Source: CAD feature listing. Evaluate the final solid. Frame: model axes, mm. Face numbers are marked on the shaded views. A direction names the side the tool comes from. Coordinates: 2 decimals unless noted, no trailing zeros. Loops run counter-clockwise (first coordinate to the right, second up) from the corner with the lowest first, then second, coordinate; pieces in that order, holes last.
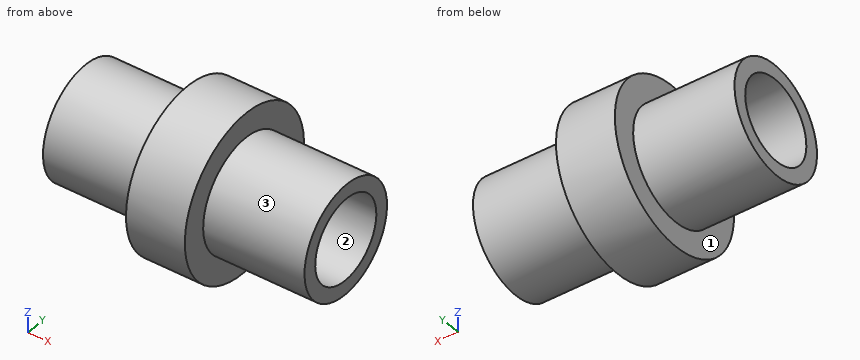
```python
from build123d import *

# Parameters (mm, degrees)
CUT_EXTRUDE1_DEPTH      = 44.767370257
CUT_EXTRUDE1_DEPTH_BACK = 44.767370257
SKETCH3_R               = 6.35


with BuildPart() as part:
    # Sketch2 → Revolve1 (revolve)
    with BuildSketch(Plane(origin=(0, 0, 0), x_dir=(1, 0, 0), z_dir=(0, 1, 0))):
        Polygon((-20.055735381, 8.5725), (-4.510240996, 8.5725), (-4.510240996, 12.3825), (4.510240996, 12.3825), (4.510240996, 8.5725), (20.055735381, 8.5725), (20.055735381, 0), (-20.055735381, 0), align=None)
    revolve(axis=Axis((20.055735381, 0, 0), (-1, 0, 0)))

    # Sketch3 → Cut-Extrude1 (cut, two sides: drawn at the far end of the back side and taken through both)
    with BuildSketch(Plane(origin=(20.055735381, 0, 0), x_dir=(0, 0, -1), z_dir=(1, 0, 0)).offset(-CUT_EXTRUDE1_DEPTH_BACK)):
        Circle(SKETCH3_R)
    extrude(amount=CUT_EXTRUDE1_DEPTH + CUT_EXTRUDE1_DEPTH_BACK, mode=Mode.SUBTRACT)


solid = part.part
```
Q1. First-contact query: pin 1 Ø3 at (x, y) = (14.5, -2.5) entering from +Z; pin 2 Ø10 at (x, z) = (-7, 8) entering from +Y; pin 3 Ø7.5 at (y, z) = (-5, -0.5) entering from -X; pin 4 Ø6 at (x, z) = (-12, -6.5) entering from -Y. Flat tips, straight axial feed; report the tip coordinate or a pass-through.
Q2. Section query A-A on y = 0. Return the cut outline in (x, z), then the cut area to 3 significant figures.
Q3. Material intervals for line 1 along Z through (x, y) = (-9, 0); line 2 along Y through (x, z) = (-1, 0), sorted ascending.
Q4. Section query D-D on y = 8. Return the cut outline in (x, z), then the cut area to 3 significant figures.
Q5. Reachability of the marked faces 1, 2 and 3 from +Z, -Z, +X, -X, +Y, -Y: full face, straight path, thin tool, end or side. Return the list, or none.
Resolved:
1. pin 1: stops at z = 8.51
1. pin 2: stops at y = 11.83
1. pin 3: stops at x = -20.06
1. pin 4: stops at y = -7.83
2. outline: (-20.06, -8.57) - (-4.51, -8.57) - (-4.51, -12.38) - (4.51, -12.38) - (4.51, -8.57) - (20.06, -8.57) - (20.06, -6.35) - (-20.06, -6.35) - close; (-20.06, 6.35) - (20.06, 6.35) - (20.06, 8.57) - (4.51, 8.57) - (4.51, 12.38) - (-4.51, 12.38) - (-4.51, 8.57) - (-20.06, 8.57) - close
2. area: 247 mm2
3. line 1: z = -8.57 to -6.35, 6.35 to 8.57
3. line 2: y = -12.38 to -6.35, 6.35 to 12.38
4. outline: (-20.06, -3.08) - (-4.51, -3.08) - (-4.51, -9.45) - (4.51, -9.45) - (4.51, -3.08) - (20.06, -3.08) - (20.06, 3.08) - (4.51, 3.08) - (4.51, 9.45) - (-4.51, 9.45) - (-4.51, 3.08) - (-20.06, 3.08) - close
4. area: 362 mm2
5. face 1: -X
5. face 2: +X, -X
5. face 3: +X
